```python
from build123d import *

# Parameters (mm, degrees)
BOSS_EXTRUDE3_START = 25
BOSS_EXTRUDE3_DEPTH = 25


# Read off the part's stored shape, not the designer's step: Revolve1
with BuildPart() as part:
    # Revolve1 outline → Revolve1 (revolve)
    with BuildSketch(Plane.XY):
        with BuildLine():
            add(Edge.make_bspline(
                [(0, -83.170194275), (9.196233186, -29.383544719), (56.312104062, -30.117818032), (14.458525258, -24.733147074), (13.097094087, -14.008197046), (13.097094087, 16.829805725)],
                knots=[0, 0, 0, 0, 0, 0, 1, 1, 1, 1, 1, 1], degree=5))
            Line((13.097094087, 16.829805725), (13.097094087, 41.829805725))
            Line((13.097094087, 41.829805725), (0, 41.829805725))
            Line((0, 41.829805725), (0, -83.170194275))
        make_face()
    revolve(axis=Axis((0, 0, 0), (0, 1, 0)))

    # Sketch5 → Boss-Extrude3 (add)
    with BuildSketch(Plane(origin=(0, 16.829805725, 0), x_dir=(1, 0, 0), z_dir=(0, 1, 0)).offset(BOSS_EXTRUDE3_START)):
        with BuildLine():
            Line((-30.925152295, -22.466241313), (-35.69384323, -13.676498042))
            Line((-35.69384323, -13.676498042), (-13.024433115, -1.377684848))
            ThreePointArc((-13.024433115, -1.377684848), (-11.512009462, -6.245599384), (-8.255742181, -10.167428119))
            Line((-8.255742181, -10.167428119), (-30.925152295, -22.466241313))
        make_face()
        with BuildLine():
            Line((29.691116354, -24.073525975), (34.918911852, -15.548846847))
            Line((34.918911852, -15.548846847), (12.933122133, -2.065968396))
            ThreePointArc((12.933122133, -2.065968396), (11.164852459, -6.846892951), (7.705326635, -10.590647524))
            Line((7.705326635, -10.590647524), (29.691116354, -24.073525975))
        make_face()
        with BuildLine():
            Line((6.002726876, 37.750024016), (5.319106481, 11.968332372))
            ThreePointArc((5.319106481, 11.968332372), (0.347157002, 13.092492335), (-4.677379952, 12.233396515))
            Line((-4.677379952, 12.233396515), (-3.993759557, 38.01508816))
            Line((-3.993759557, 38.01508816), (6.002726876, 37.750024016))
        make_face()
    extrude(amount=-BOSS_EXTRUDE3_DEPTH)


solid = part.part
```
Can you work these out from the model? Positions are in its coordinate system, mm. A direction names the side the tool comes from. Give positions to 0.01 mm unless a question says otherwise; leave off trailing zeros. Loops run counter-clockwise (first coordinate to the right, second up) from the corner with the lowest first, then second, coordinate; pieces in that order, holes last. Notation, with made-up numbers: M -26.5,61.5 L -22.5,61.5 A22 cw -22.5,70.5 Z; hole C 48,63 d1. An arc over 180 degrees is marked long. One line per question, with ' | ' between items. Start each with the question number.
Q1. If we mould it in two halves opening along Y, with no side actions, what happens to faces 1 (the flat face through (21, 16.83, 13)), 2 (the flat face through (-22, 16.83, 12)), 3 (the flat face through (2, 41.83, -3)), 4 (the flat face through (32.27, 29.5, 19.87))? For each: +Y half, -Y half, draft (parallel to the pull), parting line (faces both ways), or undercut.
Q2. If we section it at A-A (z = 17): State how many separate pieces and enclosed holes the cut face has, plus the area to 3 significant figures.
Q3. If we section it at B-B (z = -32.5): Please give me the cut outline in (x, y), plus the area to 3 significant figures.
Q4. For faces 5 (the flat face through (-33.276, 29.505, 18.133)), 6 (the flat face through (18.544, 29.505, 17.238)), which set-ups out of +Z, -Z, +X, -X, +Y, -Y let a thin tool reach every point of the face, with its end or its side?
Q5. For pin 1 Ø6 at (x, y) = (4.5, -58.5) entering from -Z; pin 2 Ø6 at (x, y) = (21, 26.5) entering from -Z; pin 3 Ø6 at (x, y) = (14.5, 23) entering from +Z, each with a flat end and sliding along its axis, tell me the tip position at first contact or that it passes through.
Q6. If I drill on line 1 (Y direction, x = 2.5, z = -23.5); line 2 (X direction, y = -12.5, z = 11.5); line 3 (Y direction, x = 15, z = 15.5), over which ranges is the centre line in solid material (lowest first)? Write a range as from..to.
Computed:
1) face 1: undercut | face 2: undercut | face 3: +Y half | face 4: draft
2) separate pieces: 3 | enclosed holes: 0 | area: 1,700 mm²
3) outline: M -4.14,16.83 L 5.86,16.83 L 5.86,41.83 L -4.14,41.83 Z | area: 250 mm²
4) face 5: +Z, -X, +Y, -Y | face 6: +Z, +Y
5) pin 1: stops at z = -9.66 | pin 2: stops at z = 5.17 | pin 3: stops at z = 16.6
6) line 1: y = -36.57..-21.71, 16.83..41.83 | line 2: x = -13.58..13.58 | line 3: y = -39.5..-18.72
